```python
from build123d import *

# Parameters (mm, degrees)
SKETCH1_W           = 80
SKETCH1_H           = 30
SKETCH1_W_2         = 50
BOSS_EXTRUDE1_DEPTH = 1.6
FILLET1_SIZE        = 60
SKETCH6_W           = 80
SKETCH6_H           = 30
CUT_EXTRUDE1_DEPTH  = 10
FILLET3_R           = 20
CUT_EXTRUDE3_REACH  = 256.563
CUT_EXTRUDE5_REACH  = 256.563
SKETCH11_R          = 1.55


with BuildPart() as part:
    # Sketch1 → Boss-Extrude1 (new body)
    with BuildSketch(Plane(origin=(0, 0, 0), x_dir=(1, 0, 0), z_dir=(0, 1, 0))):
        with Locations((-90, -15)):
            Rectangle(SKETCH1_W, SKETCH1_H)
        Polygon((0, 180), (-180, 180), (-180, 30), (-130, 30), (-50, 30), (0, 30), align=None)
        with Locations((-25, 15)):
            Rectangle(SKETCH1_W_2, SKETCH1_H)
        with Locations((-155, 15)):
            Rectangle(SKETCH1_W_2, SKETCH1_H)
        with Locations((-90, 15)):
            Rectangle(SKETCH1_W, SKETCH1_H)
    extrude(amount=BOSS_EXTRUDE1_DEPTH)

    # Fillet1
    # a fillet whose section is not a circle: 60 mm, written as the material it takes off along each edge
    with BuildSketch(Plane(origin=(0, -150, -180), x_dir=(0, 0, 1), z_dir=(0, 1, 0)), Plane(origin=(-180, -150, -180), x_dir=(1, 0, 0), z_dir=(0, 1, 0))) as fillet1_piece_1:
        with BuildLine():
            Bezier((FILLET1_SIZE, 0), (0, 0), (0, -FILLET1_SIZE), weights=[1, 0.25, 1])
            Line((0, -FILLET1_SIZE), (0, 0))
            Line((0, 0), (FILLET1_SIZE, 0))
        make_face()
    extrude(amount=301.6, mode=Mode.SUBTRACT)

    # Sketch6 → Cut-Extrude1 (cut)
    with BuildSketch(Plane(origin=(0, 1.6, 0), x_dir=(1, 0, 0), z_dir=(0, 1, 0))):
        with Locations((-90, -15)):
            Rectangle(SKETCH6_W, SKETCH6_H)
        Polygon((-180, 100), (-180, 0), (-175, 30.1112758), (-175, 67.7112758), align=None)
        Polygon((-5, 30.1112758), (0, 0), (0, 100), (-5, 67.7112758), align=None)
    extrude(amount=-CUT_EXTRUDE1_DEPTH, mode=Mode.SUBTRACT)

    # Fillet2
    # a fillet whose section is not a circle: 10 mm, written as the material it takes off along each edge
    with BuildSketch(Plane(origin=(-180, -29.493585843, 0), x_dir=(1, 0, 0), z_dir=(0, 1, 0)), Plane(origin=(0, -29.493585843, 0), x_dir=(-0.16380778451733694, 0, -0.9864922755559323), z_dir=(0, 1, 0))) as fillet2_piece_1:
        with BuildLine():
            Bezier((11.797434337, 0), (0, 0), (1.932511582, 11.638077845), weights=[1, 0.333333333, 1])
            Line((1.932511582, 11.638077845), (0, 0))
            Line((0, 0), (11.797434337, 0))
        make_face()
    extrude(amount=60.587171687, mode=Mode.SUBTRACT)

    # Fillet3
    fillet3_edges = [part.edges().sort_by_distance(p)[0] for p in [
        (0, 0.8, -100),
        (-180, 0.8, -100),
    ]]
    fillet(fillet3_edges, radius=FILLET3_R)

    # Sketch9 → Cut-Extrude3 (cut, up to next)
    with BuildSketch(Plane(origin=(0, 1.6, 0), x_dir=(1, 0, 0), z_dir=(0, 1, 0)), mode=Mode.PRIVATE) as cut_extrude3_sk1:
        Polygon((-164, 115.6), (-164, 67.6), (-16, 67.6), (-8, 101.53935467), (-8, 115.6), align=None)
    cut_extrude3_tool1 = extrude(cut_extrude3_sk1.sketch, amount=-CUT_EXTRUDE3_REACH, mode=Mode.PRIVATE) & part.part
    add(cut_extrude3_tool1.solids().sort_by_distance((-87.391012, 1.6, -91.83426))[0], mode=Mode.SUBTRACT)

    # Sketch11 → Cut-Extrude5 (cut, up to next)
    with BuildSketch(Plane(origin=(0, 1.6, 0), x_dir=(1, 0, 0), z_dir=(0, 1, 0)), mode=Mode.PRIVATE) as cut_extrude5_sk1:
        with Locations(Location((-165, 12, 0), (0, 0, 270))):
            Circle(SKETCH11_R)
    cut_extrude5_tool1 = extrude(cut_extrude5_sk1.sketch, amount=-CUT_EXTRUDE5_REACH, mode=Mode.PRIVATE) & part.part
    # Sketch11 → Cut-Extrude5 (cut, up to next)
    with BuildSketch(Plane(origin=(0, 1.6, 0), x_dir=(1, 0, 0), z_dir=(0, 1, 0)), mode=Mode.PRIVATE) as cut_extrude5_sk2:
        with Locations(Location((-126.25, 145, 0), (0, 0, 270))):
            Circle(SKETCH11_R)
    cut_extrude5_tool2 = extrude(cut_extrude5_sk2.sketch, amount=-CUT_EXTRUDE5_REACH, mode=Mode.PRIVATE) & part.part
    # Sketch11 → Cut-Extrude5 (cut, up to next)
    with BuildSketch(Plane(origin=(0, 1.6, 0), x_dir=(1, 0, 0), z_dir=(0, 1, 0)), mode=Mode.PRIVATE) as cut_extrude5_sk3:
        with Locations(Location((-15, 12, 0), (0, 0, 270))):
            Circle(SKETCH11_R)
    cut_extrude5_tool3 = extrude(cut_extrude5_sk3.sketch, amount=-CUT_EXTRUDE5_REACH, mode=Mode.PRIVATE) & part.part
    # Sketch11 → Cut-Extrude5 (cut, up to next)
    with BuildSketch(Plane(origin=(0, 1.6, 0), x_dir=(1, 0, 0), z_dir=(0, 1, 0)), mode=Mode.PRIVATE) as cut_extrude5_sk4:
        with Locations(Location((-53.75, 145, 0), (0, 0, 270))):
            Circle(SKETCH11_R)
    cut_extrude5_tool4 = extrude(cut_extrude5_sk4.sketch, amount=-CUT_EXTRUDE5_REACH, mode=Mode.PRIVATE) & part.part
    add(cut_extrude5_tool1.solids().sort_by_distance((-165, 1.6, -12))[0], mode=Mode.SUBTRACT)
    add(cut_extrude5_tool2.solids().sort_by_distance((-126.25, 1.6, -145))[0], mode=Mode.SUBTRACT)
    add(cut_extrude5_tool3.solids().sort_by_distance((-15, 1.6, -12))[0], mode=Mode.SUBTRACT)
    add(cut_extrude5_tool4.solids().sort_by_distance((-53.75, 1.6, -145))[0], mode=Mode.SUBTRACT)


solid = part.part
```
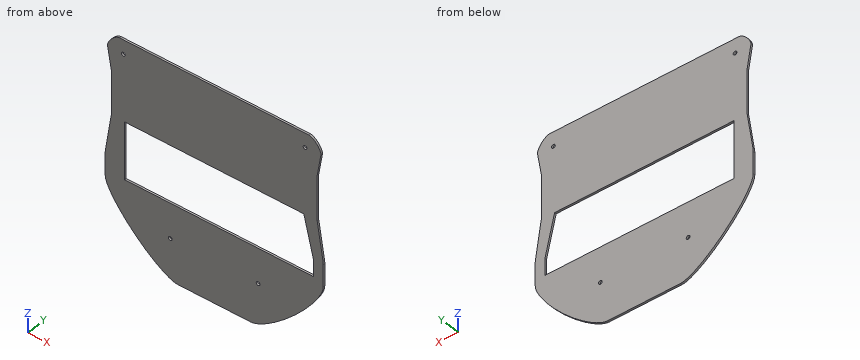
Work out the finished part from the listing and answer in its coordinate system (mm). Coordinates: 2 decimals unless noted, no trailing zeros. Write each loop counter-clockwise with the first axis right and the second up, starting at its lowest first coordinate (ties: lowest second). Pieces come first, ordered by that corner, then holes.
Q1. Find the intervals of material crossed by line 1 (Z direction, x = -85.5, y = 0.1); line 2 (X direction, y = 0.65, z = -145); line 3 (Z direction, x = -126.25, y = 0.5), in increasing order.
Q2. Each of these flat-tipped pins is pushed along its axis until it touches: pin 1 Ø0.8 at (y, z) = (0.5, -40.5) entering from +X; pin 2 Ø0.5 at (y, z) = (0.5, -94) entering from +X. Where does it stop, or does it pass through?
Q3. A cutting plane is placed at D-D, the plane y = 1.3. State how many separate pieces and enclosed holes the cut face has, then the cut area to 3 significant figures.
Q4. A cutting plane is placed at C-C, the plane z = -47. Give the vertices of the cut face in (x, y), then the cut area to 3 significant figures.
Q5. A cutting plane is placed at A-A, the plane x = -68. Give the vertices of the cut face in (y, z), then the cut area to 3 significant figures.
Q6. A cutting plane is placed at B-B, the plane z = -73.5. Give the vertices of the cut face in (x, y), then the cut area to 3 significant figures.
Findings below:
1. line 1: z = -180 to -115.6, -67.6 to 0
1. line 2: x = -166.05 to -127.8, -124.7 to -55.3, -52.2 to -13.95
1. line 3: z = -178.39 to -146.55, -143.45 to -115.6, -67.6 to 0
2. pin 1: stops at x = -5
2. pin 2: stops at x = -0.89
3. separate pieces: 1
3. enclosed holes: 5
3. area: 21,700 mm2
4. outline: (-175, 0) - (-5, 0) - (-5, 1.6) - (-175, 1.6) - close
4. area: 272 mm2
5. outline: (0, -180) - (1.6, -180) - (1.6, -115.6) - (0, -115.6) - close; (0, -67.6) - (1.6, -67.6) - (1.6, 0) - (0, 0) - close
5. area: 211 mm2
6. outline: (-175.9, 0) - (-164, 0) - (-164, 1.6) - (-175.9, 1.6) - close; (-14.61, 0) - (-4.1, 0) - (-4.1, 1.6) - (-14.61, 1.6) - close
6. area: 35.8 mm2
